Geometry: final body of the model. Coordinates: model frame, mm. Coordinates: 2 decimals unless noted, no trailing zeros. Write each loop counter-clockwise with the first axis right and the second up, starting at its lowest first coordinate (ties: lowest second). Pieces come first, ordered by that corner, then holes. Notation, with made-up numbers: M 3,71 L 10,71 A25 ccw 10,101 Z; hole C -2,2.5 d2. An arc over 180 degrees is marked long. Write item = value, one per line. Start each with the question number.
Item 1: Section D-D on x = 105. Output: boundary loops of the cut face in (y, z), plus the area to 3 significant figures.
Item 2: Ray query, L1, parallel to X at y = 9.4, z = 0; L2, parallel to Z at x = 0, y = 8.3; L3, parallel to Y at x = 0, z = -9.5. Return the intervals inside material, ascending. Write a range as [from, to].
Item 3: First-contact query: pin 1 Ø2.5 at (x, y) = (0, 3.3) entering from +Z; pin 2 Ø25 at (x, z) = (92.5, -8) entering from -Y; pin 3 Ø12 at (x, y) = (-0.5, 13.5) entering from +Z; pin 4 Ø1.7 at (x, z) = (0, 12) entering from -Y. Flat tips, straight axial feed; report the tip coordinate or a pass-through.
Item 4: Section C-C on y = 15. Output: boundary loops of the cut face in (x, z), plus the area to 3 significant figures.
Item 5: Section A-A on y = 3.3. Output: boundary loops of the cut face in (x, z), plus the area to 3 significant figures.
Item 6: Section B-B on x = 60. Output: boundary loops of the cut face in (y, z), plus the area to 3 significant figures.
from build123d import *

# Parameters (mm, degrees)
SKETCH_1_R          = 12.5
SKETCH_1_R_2        = 3.05
EXTRUDE_1_DEPTH     = 8
SKETCH_2_R          = 1.6
CUT_EXTRUDE_4_DEPTH = 12.5
SKETCH_3_R          = 4.1
SKETCH_3_R_2        = 2.1
EXTRUDE_2_DEPTH     = 4
SKETCH_4_R          = 18
EXTRUDE_3_DEPTH     = 2
FILLET_2_R          = 40
FILLET_1_R          = 1
EXTRUDE_4_DEPTH     = 10
FILLET_3_R          = 4
SKETCH_6_R          = 3.05
CUT_EXTRUDE_5_DEPTH = 12
CUT_EXTRUDE_6_REACH = 157.605


with BuildPart() as part:
    # 草图1 → 凸台-拉伸1 (new body)
    with BuildSketch(Plane(origin=(0, 0, 0), x_dir=(1, 0, 0), z_dir=(0, 1, 0))):
        with Locations(Location((0, 0, 0), (0, 0, 270))):
            Circle(SKETCH_1_R)
        with Locations(Location((0, 0, 0), (0, 0, 270))):
            Circle(SKETCH_1_R_2, mode=Mode.SUBTRACT)
    extrude(amount=EXTRUDE_1_DEPTH)

    # 草图2 → 切除-拉伸4 (cut, symmetric)
    with BuildSketch(Plane.XY):
        with Locations((0, 3.3)):
            Circle(SKETCH_2_R)
    extrude(amount=CUT_EXTRUDE_4_DEPTH, both=True, mode=Mode.SUBTRACT)

    # 草图3 → 凸台-拉伸2 (add)
    with BuildSketch(Plane(origin=(0, 8, 0), x_dir=(1, 0, 0), z_dir=(0, 1, 0))):
        with BuildLine():
            Line((2.321428571, 24.891986047), (141.114285714, 11.948153303))
            ThreePointArc((141.114285714, 11.948153303), (151.998605375, 0.182945465), (141.478035479, -11.908627592))
            Line((141.478035479, -11.908627592), (36, -25))
            Line((36, -25), (0, -25))
            ThreePointArc((0, -25), (-24.972981912, 1.161970054), (2.321428571, 24.891986047))
        make_face()
        with Locations(Location((140, 0, 0), (0, 0, 270))):
            Circle(SKETCH_3_R, mode=Mode.SUBTRACT)
        with Locations(Location((60, 0, 0), (0, 0, 270))):
            Circle(SKETCH_3_R_2, mode=Mode.SUBTRACT)
    extrude(amount=EXTRUDE_2_DEPTH)

    # 草图4 → 凸台-拉伸3 (add)
    with BuildSketch(Plane.XZ.offset(-8)):
        with Locations(Location((0, 0, 0), (0, 0, 270))):
            Circle(SKETCH_4_R)
    extrude(amount=EXTRUDE_3_DEPTH)

    # 圆角2
    fillet_2_edges = [part.edges().sort_by_distance(p)[0] for p in [
        (36, 10, 25),
    ]]
    fillet(fillet_2_edges, radius=FILLET_2_R)

    # 圆角1
    fillet_1_edges = [part.edges().sort_by_distance(p)[0] for p in [
        (0, 6, 18),
    ]]
    fillet(fillet_1_edges, radius=FILLET_1_R)

    # 草图5 → 凸台-拉伸4 (add)
    with BuildSketch(Plane(origin=(0, 12, 0), x_dir=(1, 0, 0), z_dir=(0, 1, 0))):
        with BuildLine():
            Line((0, 0), (-25, 0))
            ThreePointArc((-25, 0), (-23.096988313, -9.567085809), (-17.67766953, -17.67766953))
            Line((-17.67766953, -17.67766953), (0, 0))
        make_face()
    extrude(amount=EXTRUDE_4_DEPTH)

    # 圆角3
    fillet_3_edges = [part.edges().sort_by_distance(p)[0] for p in [
        (0, 17, 0),
    ]]
    fillet(fillet_3_edges, radius=FILLET_3_R)

    # 草图6 → 切除-拉伸5 (cut)
    with BuildSketch(Plane.XZ):
        with Locations(Location((0, 0, 0), (0, 0, 270))):
            Circle(SKETCH_6_R)
    extrude(amount=-CUT_EXTRUDE_5_DEPTH, mode=Mode.SUBTRACT)

    # 切除-拉伸6: up to this face of the body (flat: up to its plane)
    cut_extrude_6_end = Plane(part.part.faces().sort_by_distance((0, 6, 16.519167389))[0])
    # 草图7 → 切除-拉伸6 (cut, up to the picked face)
    with BuildSketch(Plane.XZ, mode=Mode.PRIVATE) as cut_extrude_6_sk1:
        with BuildLine():
            ThreePointArc((5.937171044, 11), (0, 12.5), (-5.937171044, 11))
            Line((-5.937171044, 11), (5.937171044, 11))
        make_face()
    cut_extrude_6_tool1 = split(extrude(cut_extrude_6_sk1.sketch, amount=-CUT_EXTRUDE_6_REACH, mode=Mode.PRIVATE), bisect_by=cut_extrude_6_end, keep=Keep.BOTH, mode=Mode.PRIVATE)
    # 草图7 → 切除-拉伸6 (cut, up to the picked face)
    with BuildSketch(Plane.XZ, mode=Mode.PRIVATE) as cut_extrude_6_sk2:
        with BuildLine():
            Line((5.937171044, -11), (-5.937171044, -11))
            ThreePointArc((-5.937171044, -11), (0, -12.5), (5.937171044, -11))
        make_face()
    cut_extrude_6_tool2 = split(extrude(cut_extrude_6_sk2.sketch, amount=-CUT_EXTRUDE_6_REACH, mode=Mode.PRIVATE), bisect_by=cut_extrude_6_end, keep=Keep.BOTH, mode=Mode.PRIVATE)
    add(cut_extrude_6_tool1.solids().sort_by(Axis((0, 0, 11.603197), (0, 1, 0)))[0], mode=Mode.SUBTRACT)
    add(cut_extrude_6_tool2.solids().sort_by(Axis((0, 0, -11.603197), (0, 1, 0)))[0], mode=Mode.SUBTRACT)


solid = part.part
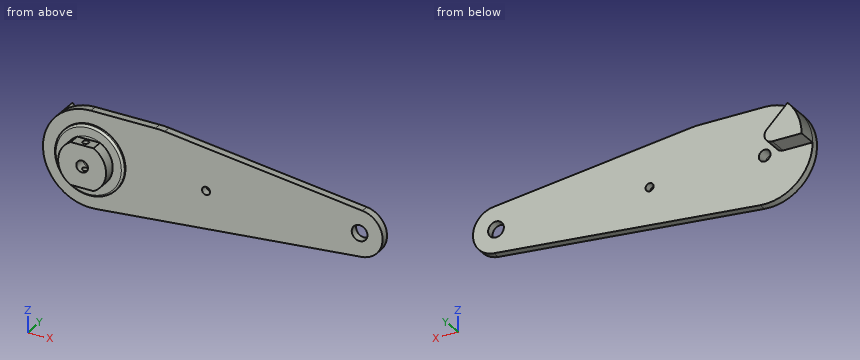
Responses:
q1.outline = M 8,-15.32 L 12,-15.32 L 12,16.44 L 8,16.44 Z
q1.area = 127 mm²
q2.L1 = [-25, -3.05], [3.05, 57.9], [62.1, 135.9], [144.1, 152]
q2.L2 = [-25, -3.05], [3.05, 25]
q2.L3 = [0, 1.7], [4.9, 12]
q3.pin_1 = through
q3.pin_2 = 8
q3.pin_3 = 25
q3.pin_4 = 6
q4.outline = M -25,0 L -9.66,0 A4 ccw -6.83,6.83 L -17.68,17.68 A25 ccw Z
q4.area = 226 mm²
q5.outline = M -5.94,-11 L -1.6,-11 L -1.6,-2.6 A3.05 cw -1.6,2.6 L -1.6,11 L -5.94,11 A12.5 ccw Z; M 1.6,-11 L 5.94,-11 A12.5 ccw 5.94,11 L 1.6,11 L 1.6,2.6 A3.05 cw 1.6,-2.6 Z
q5.area = 386 mm²
q6.outline = M 8,-19.51 L 12,-19.51 L 12,-2.1 L 8,-2.1 Z; M 8,2.1 L 12,2.1 L 12,22.02 L 8,22.02 Z
q6.area = 149 mm²
